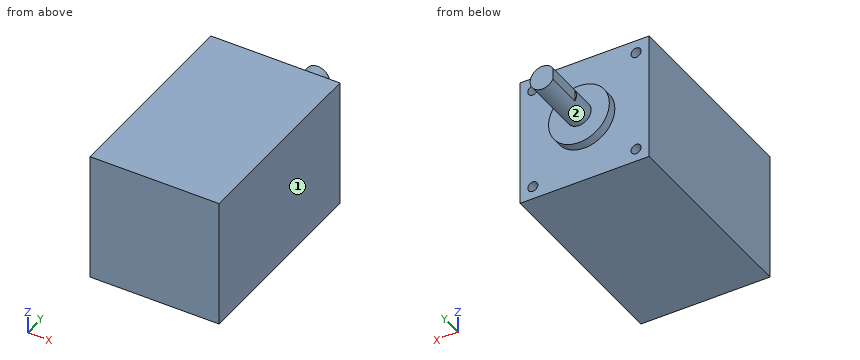
from build123d import *

# Parameters (mm, degrees)
SKETCH_1_W          = 42.5
SKETCH_1_H          = 42.5
EXTRUDE_1_DEPTH     = 65.95
SKETCH_2_R          = 10
EXTRUDE_2_DEPTH     = 3
SKETCH_3_R          = 4
EXTRUDE_3_DEPTH     = 20
HOLE_WIZARD_3_D     = 3.3
HOLE_WIZARD_3_DEPTH = 11.5
HOLE_WIZARD_3_TIP   = 0.991420021
EXTRUDE_4_DEPTH     = 12


with BuildPart() as part:
    # 스케치1 → 돌출1 (new body)
    with BuildSketch(Plane(origin=(0, 0, 0), x_dir=(-1, 0, 0), z_dir=(0, 1, 0))):
        with Locations((21.25, -21.25)):
            Rectangle(SKETCH_1_W, SKETCH_1_H)
    extrude(amount=EXTRUDE_1_DEPTH)

    # 스케치2 → 돌출2 (add)
    with BuildSketch(Plane(origin=(0, 65.95, 0), x_dir=(-1, 0, 0), z_dir=(0, 1, 0))):
        with Locations((21.25, -21.25)):
            Circle(SKETCH_2_R)
    extrude(amount=EXTRUDE_2_DEPTH)

    # 스케치3 → 돌출3 (add)
    with BuildSketch(Plane(origin=(0, 68.95, 0), x_dir=(-1, 0, 0), z_dir=(0, 1, 0))):
        with Locations((21.25, -21.25)):
            Circle(SKETCH_3_R)
    extrude(amount=EXTRUDE_3_DEPTH)

    # 구멍3
    with Locations(Plane(origin=(0, 65.95, 0), x_dir=(1, 0, 0), z_dir=(0, 1, 0))):
        with Locations((-4.25, 38.25), (-4.25, 4.25), (-38.25, 4.25), (-38.25, 38.25)):
            Hole(HOLE_WIZARD_3_D / 2, depth=HOLE_WIZARD_3_DEPTH)
            with Locations((0, 0, -(HOLE_WIZARD_3_DEPTH + HOLE_WIZARD_3_TIP / 2))):  # 118° drill point
                Cone(0, HOLE_WIZARD_3_D / 2, HOLE_WIZARD_3_TIP, mode=Mode.SUBTRACT)

    # 스케치6 → 돌출4 (cut)
    with BuildSketch(Plane(origin=(0, 88.95, 0), x_dir=(-1, 0, 0), z_dir=(0, 1, 0))):
        with BuildLine():
            Line((24.75, -19.313508327), (24.75, -23.186491673))
            ThreePointArc((24.75, -23.186491673), (25.25, -21.25), (24.75, -19.313508327))
        make_face()
    extrude(amount=-EXTRUDE_4_DEPTH, mode=Mode.SUBTRACT)


solid = part.part
Can you work these out from the model? Positions are in its coordinate system, mm. Face numbers are marked on the shaded views. A direction names the side the tool comes from. Give positions to 0.01 mm unless a question says otherwise; leave off trailing zeros. Order: outer loops, then holes, each group sorted by start corner. A loop starts at its lowest first (then second) coordinate and runs counter-clockwise, first axis right, second up. Notation, with made-up numbers: M -38,19.25 L -23,19.25 A26 ccw -23,39.25 Z; hole C 25.5,-25 d2. An arc over 180 degrees is marked long. Use a Markdown table: item, result. Add a question column.
Item 1: Will these pins go through, and if not, where does the flat tip stop? pin 1 (4.5 mm diameter, centred on y = 82.5, z = -22, fed in from -X); pin 2 (4.5 mm diameter, centred on x = -4.25, z = -38.25, fed in from +Y).
Item 2: If I drill on L1, parallel to Z at x = -4.25, y = 58.5; L2, parallel to Y at x = -30, z = -5, over which ranges is the centre line in solid material (lowest first)? Write a range as [from, to].
Item 3: Suppose I cut it at D-D (z = -27). List the corners of the cut face in (x, y) for me, then the cut area to 3 significant figures.
Item 4: Suppose I cut it at A-A (x = -21.25). List the corners of the cut face in (y, z) for me, then the cut area to 3 significant figures.
Item 5: For the marked faces 1 and 2, which set-ups out of +Z, -Z, +X, -X, +Y, -Y let a thin tool reach every point of the face, with its end or its side?
Item 6: Suppose I cut it at C-C (y = 76). List the corners of the cut face in (x, z) for me, then the cut area to 3 significant figures.
Item 7: Suppose I cut it at B-B (z = -21.25). List the corners of the cut face in (x, y) for me.
Answer sheet:
| question | item | result |
|---|---|---|
| 1 | pin 1 | stops at x = -24.75 |
| 1 | pin 2 | stops at y = 65.95 |
| 2 | L1 | z = [-42.5, -39.9], [-36.6, -5.9], [-2.6, 0] |
| 2 | L2 | y = [0, 65.95] |
| 3 | outline | M -42.5,0 L 0,0 L 0,65.95 L -13.07,65.95 L -13.07,68.95 L -29.43,68.95 L -29.43,65.95 L -42.5,65.95 Z |
| 3 | area | 2,850 mm² |
| 4 | outline | M 0,-42.5 L 65.95,-42.5 L 65.95,-31.25 L 68.95,-31.25 L 68.95,-25.25 L 88.95,-25.25 L 88.95,-17.25 L 68.95,-17.25 L 68.95,-11.25 L 65.95,-11.25 L 65.95,0 L 0,0 Z |
| 4 | area | 3,020 mm² |
| 5 | face 1 | +Z, -Z, +X, +Y, -Y |
| 5 | face 2 | +Y |
| 6 | outline | C -21.25,-21.25 d8 |
| 6 | area | 50.3 mm² |
| 7 | outline | M -42.5,0 L 0,0 L 0,65.95 L -11.25,65.95 L -11.25,68.95 L -17.25,68.95 L -17.25,88.95 L -24.75,88.95 L -24.75,76.95 L -25.25,76.95 L -25.25,68.95 L -31.25,68.95 L -31.25,65.95 L -42.5,65.95 Z |
